from build123d import *

# Parameters (mm, degrees)
SKETCH1_W               = 22.35
SKETCH1_H               = 30.25
BOSS_EXTRUDE1_DEPTH     = 0.8
SKETCH2_R               = 1.075
CUT_EXTRUDE1_DEPTH      = 1.8
CUT_EXTRUDE1_DEPTH_BACK = 1.8
BOSS_EXTRUDE2_DEPTH     = 2.3
SKETCH4_W               = 8
SKETCH4_H               = 5.6
BOSS_EXTRUDE3_DEPTH     = 2.6
SKETCH5_W               = 12.7
SKETCH5_H               = 12.7
BOSS_EXTRUDE4_DEPTH     = 7.4
SKETCH6_W               = 2.75
SKETCH6_H               = 18.1
BOSS_EXTRUDE5_DEPTH     = 9


with BuildPart() as part:
    # Sketch1 → Boss-Extrude1 (new body, symmetric)
    with BuildSketch(Plane(origin=(0, 0, 0), x_dir=(1, 0, 0), z_dir=(0, 1, 0))):
        Rectangle(SKETCH1_W, SKETCH1_H)
    extrude(amount=BOSS_EXTRUDE1_DEPTH, both=True)

    # Sketch2 → Cut-Extrude1 (cut, two sides)
    with BuildSketch(Plane(origin=(0, 0, 0), x_dir=(1, 0, 0), z_dir=(0, 1, 0))) as cut_extrude1_sk:
        with Locations((8.9, 8.55)):
            Circle(SKETCH2_R)
        with Locations((8.9, -13.05)):
            Circle(SKETCH2_R)
        with Locations((-8.9, 8.55)):
            Circle(SKETCH2_R)
        with Locations((-8.9, -13.05)):
            Circle(SKETCH2_R)
    extrude(amount=CUT_EXTRUDE1_DEPTH, mode=Mode.SUBTRACT)
    extrude(cut_extrude1_sk.sketch, amount=-CUT_EXTRUDE1_DEPTH_BACK, mode=Mode.SUBTRACT)

    # Sketch3 → Boss-Extrude2 (add, symmetric)
    with BuildSketch(Plane(origin=(0, 0, 0), x_dir=(1, 0, 0), z_dir=(0, 1, 0))):
        Polygon((-10.175, 6.75), (-7.1, 6.75), (-7.1, 10.35), (-10.175, 10.35), (-10.175, 14.125), (10.175, 14.125), (10.175, 10.35), (7.1, 10.35), (7.1, 6.75), (10.175, 6.75), (10.175, -2.25), (10.175, -11.25), (7.1, -11.25), (7.1, -14.125), (-7.1, -14.125), (-7.1, -11.25), (-10.175, -11.25), (-10.175, -2.25), align=None)
    extrude(amount=BOSS_EXTRUDE2_DEPTH, both=True)

    # Sketch4 → Boss-Extrude3 (add)
    with BuildSketch(Plane(origin=(0, 0.8, 0), x_dir=(1, 0, 0), z_dir=(0, 1, 0))):
        with Locations((0, -14.325)):
            Rectangle(SKETCH4_W, SKETCH4_H)
    extrude(amount=BOSS_EXTRUDE3_DEPTH)

    # Sketch5 → Boss-Extrude4 (add)
    with BuildSketch(Plane(origin=(0, 0.8, 0), x_dir=(1, 0, 0), z_dir=(0, 1, 0))):
        with Locations((0, 8.425)):
            Rectangle(SKETCH5_W, SKETCH5_H)
    extrude(amount=BOSS_EXTRUDE4_DEPTH)

    # Sketch6 → Boss-Extrude5 (add)
    with BuildSketch(Plane(origin=(0, 0.8, 0), x_dir=(1, 0, 0), z_dir=(0, 1, 0))):
        with Locations((9.9, -2.075)):
            Rectangle(SKETCH6_W, SKETCH6_H)
    extrude(amount=BOSS_EXTRUDE5_DEPTH)


solid = part.part
Input: part model. Units: mm. Frame: model coordinates. A direction names the side the tool comes from. Give positions to 0.01 mm unless a question says otherwise; leave off trailing zeros. Write each loop counter-clockwise with the first axis right and the second up, starting at its lowest first coordinate (ties: lowest second). Pieces come first, ordered by that corner, then holes.
Q1. Section B-B, the plane x = 1.5. Output: boundary loops of the cut face in (y, z) (3 decimals), plus the area to 3 significant figures.
Q2. First-contact query: P1, Ø2, axis at y = 2.5, z = 15, coming from the -X side; P2, Ø2, axis at y = -0.5, z = 9, coming from the +X side (3 decimals); P3, Ø1.6, axis at x = 8.5, y = -1.5, coming from the +Z side (3 decimals). Flat tips, straight axial feed; report the tip coordinate or a pass-through.
Q3. Material intervals for probe 1 along X at (y, z) = (0.35, -8.55) (3 decimals); probe 2 along Z at (x, y) = (8.9, 0.25) (3 decimals); probe 3 along X at (y, z) = (3, -3) (3 decimals), sorted ascending.
Q4. Section C-C, the plane y = 7.5. Output: boundary loops of the cut face in (x, z) (3 decimals), plus the area to 3 significant figures.
Q5. Pull-direction query (Z, two-part tool) for faces 6 (the face through (9, 2, 11.25)), 7 (the face through (-9, -2, -6.75)), 8 (the face through (0, 8.2, -9)); classes: pulls with the +Z half, pulls with the -Z half, needs draft (parallel to the pull), parting line crosses it, or undercut.
Q6. Section A-A, the plane z = 13.05. Output: boundary loops of the cut face in (x, y) (3 decimals), plus the area to 3 significant figures.
Q7. Section D-D, the plane x = 8.9. State how many separate pieces and enclosed holes the cut face has, plus the area to 3 significant figures.
Q8. Set-up query: faces 1 (the face through (6, 2, 14.125)), 2 (the face through (0, -2, -14.125)), 3 (the face through (7.1, -2, 13)), 4 (the face through (10.175, 2, -12)), 5 (the face through (-10.175, 2, 2)). Return all of +Z, -Z, +X, -X, +Y, -Y with unobstructed straight access to the full face (end or side cutting, diameter ignored); none if empty.
Filled in:
1. outline: (-2.3, -14.125) - (-0.8, -14.125) - (-0.8, -15.125) - (0.8, -15.125) - (0.8, -14.775) - (8.2, -14.775) - (8.2, -2.075) - (2.3, -2.075) - (2.3, 11.525) - (3.4, 11.525) - (3.4, 17.125) - (0.8, 17.125) - (0.8, 15.125) - (-0.8, 15.125) - (-0.8, 14.125) - (-2.3, 14.125) - close
1. area: 220 mm2
2. P1: stops at x = -7.1
2. P2: stops at x = 11.175
2. P3: stops at z = 15.125
3. probe 1: x = -11.175 to -9.975, -7.825 to 7.825, 9.975 to 11.175
3. probe 2: z = -15.125 to -9.625, -7.475 to 11.975, 14.125 to 15.125
3. probe 3: x = -6.35 to 6.35, 8.525 to 11.275
4. outline: (-6.35, -14.775) - (6.35, -14.775) - (6.35, -2.075) - (-6.35, -2.075) - close; (8.525, -6.975) - (11.275, -6.975) - (11.275, 11.125) - (8.525, 11.125) - close
4. area: 211 mm2
5. face 6: pulls with the +Z half
5. face 7: undercut
5. face 8: needs draft
6. outline: (-11.175, -0.8) - (-9.975, -0.8) - (-9.975, 0.8) - (-11.175, 0.8) - close; (-7.825, -0.8) - (-7.1, -0.8) - (-7.1, -2.3) - (7.1, -2.3) - (7.1, -0.8) - (7.825, -0.8) - (7.825, 0.8) - (7.1, 0.8) - (7.1, 2.3) - (4, 2.3) - (4, 3.4) - (-4, 3.4) - (-4, 2.3) - (-7.1, 2.3) - (-7.1, 0.8) - (-7.825, 0.8) - close; (9.975, -0.8) - (11.175, -0.8) - (11.175, 0.8) - (9.975, 0.8) - close
6. area: 80.3 mm2
7. separate pieces: 3
7. enclosed holes: 0
7. area: 243 mm2
8. face 1: +Z, +X, +Y
8. face 2: -Z, +X, -X, -Y
8. face 3: +Z, +X, -Y
8. face 4: -Z, +X, +Y
8. face 5: +Z, -Z, -X, +Y
